from build123d import *

# Parameters (mm, degrees)
SKETCH1_W           = 0.635
SKETCH1_H           = 0.635
BOSS_EXTRUDE1_DEPTH = 11.157
BOSS_EXTRUDE2_DEPTH = 2.54
SKETCH3_R           = 0.254
SKETCH4_R           = 0.254
SKETCH6_R           = 0.254
BOSS_EXTRUDE3_DEPTH = 0.01
SKETCH7_R           = 0.254
BOSS_EXTRUDE4_DEPTH = 0.01


with BuildPart() as part:
    # Sketch1 → Boss-Extrude1 (new body)
    with BuildSketch(Plane.XY.offset(5.092)):
        Rectangle(SKETCH1_W, SKETCH1_H)
    extrude(amount=-BOSS_EXTRUDE1_DEPTH)

    # Sketch2 → Boss-Extrude2 (add)
    with BuildSketch(Plane.XY):
        Polygon((-1.27, 0.635), (-0.635, 1.27), (0.635, 1.27), (1.27, 0.635), (1.27, -0.635), (0.635, -1.27), (-0.635, -1.27), (-1.27, -0.635), align=None)
    extrude(amount=BOSS_EXTRUDE2_DEPTH)

    # Sketch3 → section 0 of loft1
    with BuildSketch(Plane.XY.offset(5.342), mode=Mode.PRIVATE) as loft1_s0:
        Circle(SKETCH3_R)
    # loft up to a face of the part (loft1)
    loft([loft1_s0.sketch, part.faces().sort_by_distance((0, 0, 5.092))[0]])

    # Sketch4 → section 0 of loft2
    with BuildSketch(Plane(origin=(0, 0, -6.315), x_dir=(-1, 0, 0), z_dir=(0, 0, -1)), mode=Mode.PRIVATE) as loft2_s0:
        Circle(SKETCH4_R)
    # loft up to a face of the part (loft2)
    loft([loft2_s0.sketch, part.faces().sort_by_distance((0, 0, -6.065))[0]])

    # Sketch6 → Boss-Extrude3 (add)
    with BuildSketch(Plane.XY.offset(5.342)):
        Circle(SKETCH6_R)
    extrude(amount=BOSS_EXTRUDE3_DEPTH)

    # Sketch7 → Boss-Extrude4 (add)
    with BuildSketch(Plane(origin=(0, 0, -6.315), x_dir=(-1, 0, 0), z_dir=(0, 0, -1))):
        Circle(SKETCH7_R)
    extrude(amount=BOSS_EXTRUDE4_DEPTH)


solid = part.part
The listing builds one solid part. Answer for the finished solid, in the listing's coordinates (mm). Coordinates: 2 decimals unless noted, no trailing zeros. Loops run counter-clockwise (first coordinate to the right, second up) from the corner with the lowest first, then second, coordinate; pieces in that order, holes last.
1) Flat-ended cylindrical pins translate along their axes: pin 1 Ø0.7 at (y, z) = (0, -3) entering from +X; pin 2 Ø0.5 at (y, z) = (0, -4) entering from -X; pin 3 Ø0.5 at (x, z) = (0, -2) entering from +Y; pin 4 Ø1.5 at (x, z) = (-1, 3) entering from -Y. Find the tip coordinate at first contact, or state that the pin passes through.
2) Find the intervals of material crossed by L1, parallel to Y at x = -0.1, z = -0.25; L2, parallel to Z at x = 0.3, y = -0.4, in increasing order.
3) Find section A-A on z = 0.25. Write down the section's boundary in (x, y) (3 decimals).
4) Find section B-B on x = -0.5. Write down the section's boundary in (y, z).
5) Find section C-C on y = 1.05. Write down the section's boundary in (x, z) (3 decimals).
Values:
1. pin 1: stops at x = 0.32
1. pin 2: stops at x = -0.32
1. pin 3: stops at y = 0.32
1. pin 4: stops at y = -1.27
2. L1: y = -0.32 to 0.32
2. L2: z = 0 to 2.54
3. outline: (-1.27, -0.635) - (-0.635, -1.27) - (0.635, -1.27) - (1.27, -0.635) - (1.27, 0.635) - (0.635, 1.27) - (-0.635, 1.27) - (-1.27, 0.635) - close
4. outline: (-1.27, 0) - (1.27, 0) - (1.27, 2.54) - (-1.27, 2.54) - close
5. outline: (-0.855, 0) - (0.855, 0) - (0.855, 2.54) - (-0.855, 2.54) - close
